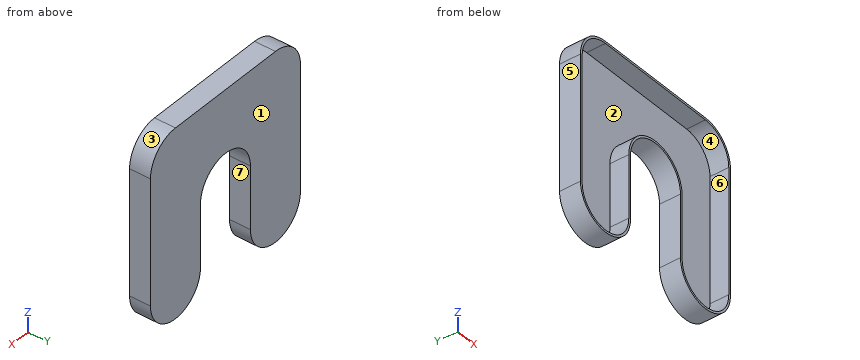
```python
from build123d import *

# Parameters (mm, degrees)
F1_DEPTH = 10
F2_T     = -1


with BuildPart() as f1:
    # F0 (on Front) → F1 (new body)
    with BuildSketch(Plane.XZ):
        with BuildLine():
            Line((30, 45), (-30, 45))
            ThreePointArc((-30, 45), (-40.606602, 40.606602), (-45, 30))
            Line((-45, 30), (-45, -30))
            ThreePointArc((-45, -30), (-30, -45), (-15, -30))
            Line((-15, -30), (-15, 0))
            ThreePointArc((-15, 0), (0, 15), (15, 0))
            Line((15, 0), (15, -30))
            ThreePointArc((15, -30), (30, -45), (45, -30))
            Line((45, -30), (45, 30))
            ThreePointArc((45, 30), (40.606602, 40.606602), (30, 45))
        make_face()
    extrude(amount=F1_DEPTH)

    # F2
    f2_openings = [f1.faces().sort_by_distance(p)[0] for p in [
        (0, -10, 43.727208),
    ]]
    offset(amount=F2_T, openings=f2_openings)


solid = f1.part
```
For this review, take the finished solid that the model builds, in its own axes (mm). Face numbers are marked on the shaded views. A direction names the side the tool comes from. Coordinates: 2 decimals unless noted, no trailing zeros. Write each loop counter-clockwise with the first axis right and the second up, starting at its lowest first coordinate (ties: lowest second). Pieces come first, ordered by that corner, then holes. Notation, with made-up numbers: (-40, 22) - (0, 22) arc R4 cw to (0, 27) - close; hole circle Ø2 at (-14.75, -37). An arc over 180 degrees is marked (long way). Answer in a Markdown table with one row per item. Add a question column.
Q1. We need section C-C, the plane x = -2.5. State the section outline as (y, z) points, and give its area (3 significant figures).
Q2. We need section D-D, the plane z = 21. State the section outline as (x, y) points, and give its area (3 significant figures).
Q3. For P1, Ø4, axis at x = -20, y = -3, coming from the -Z side; P2, Ø1, axis at x = -8.5, y = -2, coming from the -Z side, all flat-tipped, find the tip position at first contact; note any pin that passes through.
Q4. For probe 1 along X at (y, z) = (-2.5, -24); probe 2 along X at (y, z) = (-5.75, 29); probe 3 along Z at (x, y) = (0.5, -6.25), list the stretches that pass through material, from the lowest coordinate up.
Q5. Tool access review of the marked faces 5, 6 and 7: name each direction out of +Z, -Z, +X, -X, +Y, -Y from which nothing blocks a thin tool from reaching the whole face with its end or side.
Q6. Draft analysis for pull direction Z (two halves, no side actions). For the marked faces 1, 2, 3 and 4, state which applies: +Z half, -Z half, draft (parallel to the pull), parting line (faces both ways), or undercut.
Q7. We need section B-B, the plane y = -3.75. State the section outline as (x, z) points, and give its area (3 significant figures).
Q8. We need section A-A, the plane z = -10.5. State the section outline as (x, y) points, and give its area (3 significant figures).
Answer list:
| question | item | result |
|---|---|---|
| 1 | outline | (-10, 14.79) - (0, 14.79) - (0, 45) - (-10, 45) - (-10, 44) - (-1, 44) - (-1, 15.8) - (-10, 15.8) - close |
| 1 | area | 48.3 mm2 |
| 2 | outline | (-45, -10) - (-44, -10) - (-44, -1) - (44, -1) - (44, -10) - (45, -10) - (45, 0) - (-45, 0) - close |
| 2 | area | 108 mm2 |
| 3 | P1 | stops at z = -42.69 |
| 3 | P2 | stops at z = 12 |
| 4 | probe 1 | x = -45 to -44, -16 to -15, 15 to 16, 44 to 45 |
| 4 | probe 2 | x = -45 to -44, 44 to 45 |
| 4 | probe 3 | z = 14.99 to 15.99, 44 to 45 |
| 5 | face 5 | +Z, -Z, -X, +Y, -Y |
| 5 | face 6 | -Y |
| 5 | face 7 | -Z, +Y, -Y |
| 6 | face 1 | draft |
| 6 | face 2 | undercut |
| 6 | face 3 | +Z half |
| 6 | face 4 | undercut |
| 7 | outline | (-45, -30) arc R15 ccw to (-15, -30) - (-15, 0) arc R15 cw to (15, 0) - (15, -30) arc R15 ccw to (45, -30) - (45, 30) arc R15 ccw to (30, 45) - (-30, 45) arc R15 ccw to (-45, 30) - close; hole (-44, -30) arc R14 ccw to (-16, -30) - (-16, 0) arc R16 cw to (16, 0) - (16, -30) arc R14 ccw to (44, -30) - (44, 30) arc R14 ccw to (30, 44) - (-30, 44) arc R14 ccw to (-44, 30) - close |
| 7 | area | 425 mm2 |
| 8 | outline | (-45, -10) - (-44, -10) - (-44, -1) - (-16, -1) - (-16, -10) - (-15, -10) - (-15, 0) - (-45, 0) - close; (15, -10) - (16, -10) - (16, -1) - (44, -1) - (44, -10) - (45, -10) - (45, 0) - (15, 0) - close |
| 8 | area | 96.0 mm2 |
